```python
from build123d import *

# Parameters (mm, degrees)
F1_DEPTH    = 5
F2_DEPTH    = 5
F3_T2_ANGLE = 28.7632092252
F3_T4_ANGLE = 28.7632092252
F4_T1_DEPTH = 73.2511453801
F4_T4_ANGLE = 58.5309171072
F4_T6_ANGLE = 58.5309171072
F5_W        = 5
F5_H        = 30
F6_DEPTH    = 10


# Not quite as in the source:
# - a fillet or chamfer that OpenCascade refuses, or shapes differently, is made with other operations: its cross-section is extruded or revolved along the edge and cut away or added


with BuildPart() as f1:
    # F0 (on Front) → F1 (new body, symmetric)
    with BuildSketch(Plane.XZ):
        with BuildLine():
            Line((2.6443716172, -3.0652818078), (2.6443716172, -47.137426524))
            Line((2.6443716172, -47.137426524), (50, -47.137426524))
            ThreePointArc((50, -47.137426524), (128.4023811423, -29.5875675392), (191.8408584792, 19.7124376571))
            ThreePointArc((191.8408584792, 19.7124376571), (121.8130563717, 2.8164742266), (50, -2.862573476))
            Line((50, -2.862573476), (2.6443716172, -3.0652818078))
        make_face()
    extrude(amount=F1_DEPTH, both=True)

    # F0 (on Front) → F2 (join, symmetric)
    with BuildSketch(Plane.XZ):
        with BuildLine():
            Line((2.6443716172, -50), (50, -50))
            ThreePointArc((50, -50), (133.9633393999, -30.0622505081), (200, 25.494168336))
            ThreePointArc((200, 25.494168336), (127.7176805201, 6.7011176968), (53.3323914074, 0.0122294972))
            Line((53.3323914074, 0.0122294972), (50, -2.862573476))
            ThreePointArc((50, -2.862573476), (121.8130563717, 2.8164742266), (191.8408584792, 19.7124376571))
            ThreePointArc((191.8408584792, 19.7124376571), (128.4023811423, -29.5875675392), (50, -47.137426524))
            Line((50, -47.137426524), (2.6443716172, -47.137426524))
            Line((2.6443716172, -47.137426524), (2.6443716172, -50))
        make_face()
        Polygon((50, -2.862573476), (53.3323914074, 0.0122294972), (49.9881391504, -0.0917057033), align=None)
        with BuildLine():
            Line((2.6443716172, -3.0652818078), (2.6443716172, -47.137426524))
            Line((2.6443716172, -47.137426524), (50, -47.137426524))
            ThreePointArc((50, -47.137426524), (128.4023811423, -29.5875675392), (191.8408584792, 19.7124376571))
            ThreePointArc((191.8408584792, 19.7124376571), (121.8130563717, 2.8164742266), (50, -2.862573476))
            Line((50, -2.862573476), (2.6443716172, -3.0652818078))
        make_face()
    extrude(amount=F2_DEPTH, both=True)

    # F3: chamfer of 5.08 on 2 edges, made by hand

    # F3_s1 → F3_t2 (revolve, cut)
    with BuildSketch(Plane(origin=(195.1630456204, 0, 74.6833379712), x_dir=(0, 1, 0), z_dir=(0.9339525469, 0, 0.3573970343))):
        Polygon((-5, -52.9370117112), (0.08, -47.8570117112), (-5, -47.8570117112), align=None)
    revolve(axis=Axis((50, -5, 454.0244716756), (0, 1, 0)), revolution_arc=F3_T2_ANGLE, mode=Mode.SUBTRACT)

    # F3_s3 → F3_t4 (revolve, cut)
    with BuildSketch(Plane(origin=(195.1630456204, 0, 74.6833379712), x_dir=(0, 1, 0), z_dir=(0.9339525469, 0, 0.3573970343))):
        Polygon((-0.08, -47.8570117112), (5, -52.9370117112), (5, -47.8570117112), align=None)
    revolve(axis=Axis((50, 5, 454.0244716756), (0, 1, 0)), revolution_arc=F3_T4_ANGLE, mode=Mode.SUBTRACT)

    # F4: chamfer of 5.08 x 10 on 2 edges, made by hand

    # F4_s2 → F4_t1 (cut)
    with BuildSketch(Plane.YZ.offset(-23.2511453801)):
        Polygon((0.08, -50), (-5, -40), (-5, -50), align=None)
        Polygon((5, -40), (-0.08, -50), (5, -50), align=None)
    extrude(amount=F4_T1_DEPTH, mode=Mode.SUBTRACT)

    # F4_s3 → F4_t4 (revolve, cut)
    with BuildSketch(Plane.YZ.offset(50)):
        Polygon((5, -40), (-0.08, -50), (5, -50), align=None)
    revolve(axis=Axis((50, 5, 136.7652169319), (0, -1, 0)), revolution_arc=F4_T4_ANGLE, mode=Mode.SUBTRACT)

    # F4_s5 → F4_t6 (revolve, cut)
    with BuildSketch(Plane.YZ.offset(50)):
        Polygon((-5, -40), (0.08, -50), (-5, -50), align=None)
    revolve(axis=Axis((50, -5, 136.7652169319), (0, -1, 0)), revolution_arc=F4_T6_ANGLE, mode=Mode.SUBTRACT)

    # F5 (on face) → F6 (join)
    with BuildSketch(Plane(origin=(2.6443716172, 0, 0), x_dir=(0, -1, 0), z_dir=(-1, 0, 0))):
        with Locations((0, -22.5)):
            Rectangle(F5_W, F5_H)
    extrude(amount=F6_DEPTH)


solid = f1.part
```
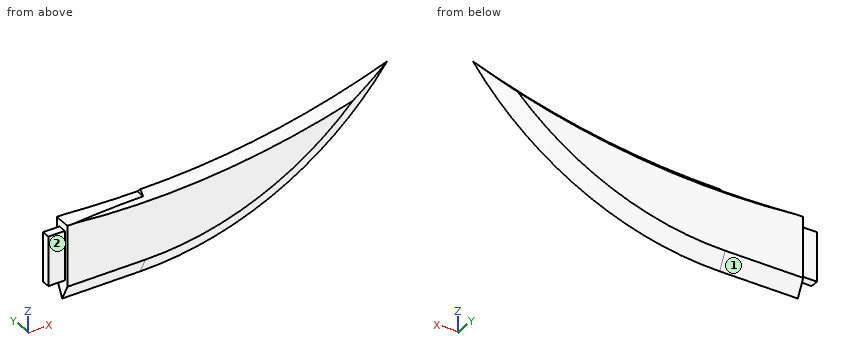
The model under review builds one solid part; all positions refer to its coordinate system, in mm. Face numbers are marked on the shaded views. A direction names the side the tool comes from. Round coordinates to 2 decimals unless told otherwise and drop trailing zeros. Answer in a Markdown table with one row per item.
(1) For line 1 (Z direction, x = 25.5, y = 2); line 2 (Z direction, x = 96, y = -4); line 3 (Y direction, x = 167, z = 14), list the stretches that pass through material, from the lowest coordinate up. Write a range as from..to.
Result set:
| item | result |
|---|---|
| line 1 | z = -45.91..-2.97 |
| line 2 | z = -35.95..-1.76 |
| line 3 | y = -1.21..1.21 |
(2) Clearance check with flat-ended pins moving along their axes: P1, Ø2.5, axis at x = -2, y = 0.5, coming from the -Z side; P2, Ø4, axis at x = 42.5, y = 2.5, coming from the -Z side; P3, Ø4, axis at x = -1.5, y = 1, coming from the +Z side. State where each tip first meets the part, or that it passes through.
Result set:
| item | result |
|---|---|
| P1 | stops at z = -37.5 |
| P2 | stops at z = -48.86 |
| P3 | stops at z = -7.5 |
(3) Machinability: for the marked faces 1 and 2, which of the approach directions +Z, -Z, +X, -X, +Y, -Y give a long, thin tool a straight path to every point of the face, cutting with its end or side? Answer none if there is none.
Result set:
| item | result |
|---|---|
| face 1 | -Z, +X, -X, +Y |
| face 2 | +Z, -Z, -X, -Y |
